Input: part model. Units: mm. Frame: model coordinates. Face numbers are marked on the shaded views. Coordinates: 2 decimals unless noted, no trailing zeros. Write each loop counter-clockwise with the first axis right and the second up, starting at its lowest first coordinate (ties: lowest second). Pieces come first, ordered by that corner, then holes. Notation, with made-up numbers: (-32.75, -9.5) -> (-17.75, -9.5) arc R17 cw to (-17.75, 0.5) -> close; hole circle Ø11 at (60.5, -10). An arc over 180 degrees is marked (long way). Use one line per item in the form item = value. Start each with the question number.
(1) First-contact query: pin 1 (4.5 mm diameter, centred on y = 12, z = 23.5, fed in from -X); pin 2 (1.5 mm diameter, centred on y = 15.5, z = 33, fed in from -X); pin 3 (4 mm diameter, centred on x = -2.5, z = 84.5, fed in from +Y); pin 4 (2 mm diameter, centred on x = 0.5, y = 2, fed in from -Z). Flat tips, straight axial feed; report the tip coordinate or a pass-through.
(2) Ray query, line 1 along X through (y, z) = (10, 23.5); line 2 along X through (y, z) = (-6.5, 5); line 3 along X through (y, z) = (6, 87.5). Return the intervals inside material, ascending.
(3) Pull-direction query (X, two-part tool) for the marked faces 1, 2 and 3; classes: released by +X, released by -X, zero draft, split by the parting line, or undercut.
(4) Cut plane D-D on z = 62. Return the cut outline in (x, y), plus the area to 3 significant figures.
(5) Cut plane A-A on z = 30. Return the cut outline in (x, y), plus the area to 3 significant figures.
```python
from build123d import *

# Parameters (mm, degrees)
F1_DEPTH = 100
F3_DEPTH = 35
F4_SIZE2 = 99.99999
F4_SIZE  = 7.49999


# Not quite as in the source:
# - a fillet or chamfer is up to 0.001 mm smaller than in the source, because OpenCascade refuses the exact size


with BuildPart() as f1:
    # F0 (on Top) → F1 (new body)
    with BuildSketch(Plane.XY):
        Polygon((-7.5, 20), (-7.5, 0), (0, -20), (7.5, 0), (7.5, 20), align=None)
    extrude(amount=F1_DEPTH)

    # F2 (on face) → F3 (cut)
    with BuildSketch(Plane(origin=(0, 0, 0), x_dir=(1, 0, 0), z_dir=(0, 0, -1))):
        Polygon((0, 8.6079950062), (-3.5, -0.7253383271), (-3.5, -16), (3.5, -16), (3.5, -0.7253383271), align=None)
    extrude(amount=-F3_DEPTH, mode=Mode.SUBTRACT)

    # F4 (size 7.5 and 100 in the source; OpenCascade refuses exactly that, so slightly less here)
    f4_edges = [f1.edges().sort_by_distance(p)[0] for p in [
        (3.75, -10, 100),
        (-3.75, -10, 100),
        (7.5, 10, 100),
        (-7.5, 10, 100),
    ]]
    f4_side = f1.faces().sort_by_distance((0, 4.444444, 100))[0]
    chamfer(f4_edges, length=F4_SIZE, length2=F4_SIZE2, reference=f4_side)


solid = f1.part
```
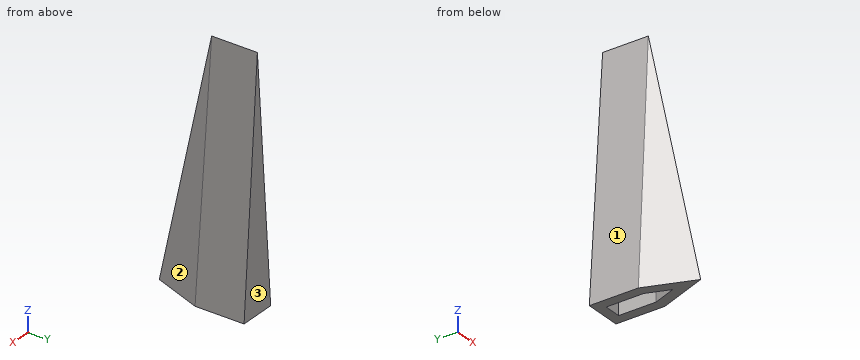
Values:
q1.pin_1 = -5.91
q1.pin_2 = -5.08
q1.pin_3 = 20
q1.pin_4 = 35
q2.line_1 = -5.74 to -3.5, 3.5 to 5.74
q2.line_2 = -4.66 to -0.79, 0.79 to 4.66
q2.line_3 = -0.94 to 0.94
q3.face_1 = released by -X
q3.face_2 = released by +X
q3.face_3 = zero draft
q4.outline = (-2.85, 0.84) -> (0, -6.76) -> (2.85, 0.84) -> (2.85, 20) -> (-2.85, 20) -> close
q4.area = 131 mm2
q5.outline = (-5.25, 0.41) -> (0, -13.59) -> (5.25, 0.41) -> (5.25, 20) -> (-5.25, 20) -> close; hole (-3.5, 0.73) -> (0, -8.61) -> (3.5, 0.73) -> (3.5, 16) -> (-3.5, 16) -> close
q5.area = 140 mm2
